Check sheet for the drawn part. Datum: minimum x, y, z corner. Units: mm. Give positions to 0.01 mm unless a question says otherwise; leave off trailing zeros. Write each loop counter-clockwise with the first axis right and the second up, starting at its lowest first coordinate (ties: lowest second). Pieces come first, ordered by that corner, then holes. Notation, with made-up numbers: (-6, 67) -> (0, 67) arc R24 ccw to (0, 102) -> close; hole circle Ø10 at (41, 49.25). An arc over 180 degrees is marked (long way). Use CSV: the item, a comma, the result in double quotes. Start each with the question number.
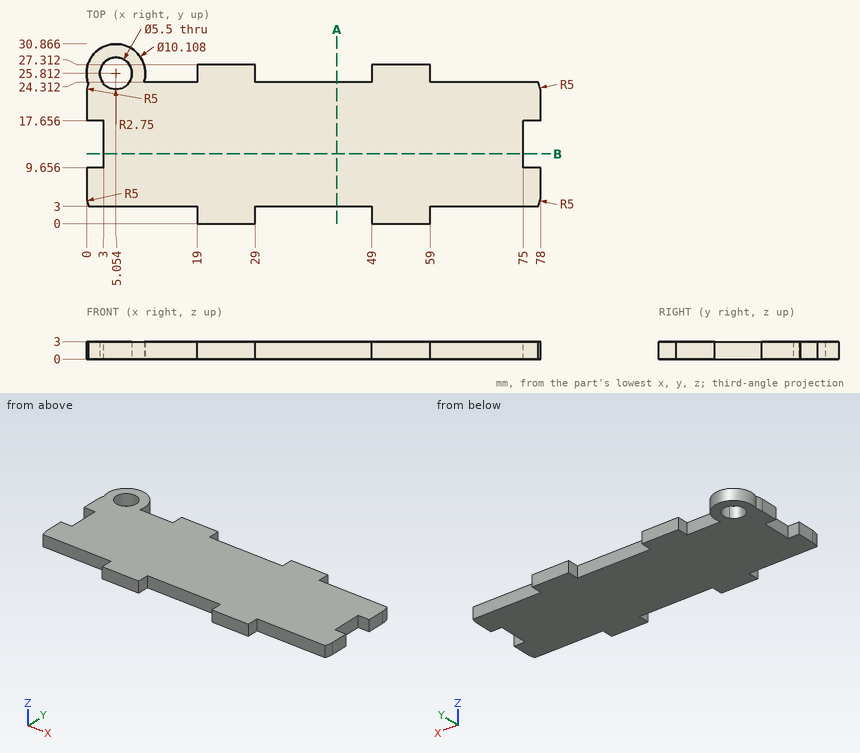
(1) Thickness scan on line 1 (Y direction, x = 64, z = 0.7); line 2 (X direction, y = 10.5, z = 1); line 3 (Y direction, x = 20, z = 0.85). Record the ranges inside material, lowest first. Write a range as from..to.
(2) Section check B-B on y = 12. Record the cut outline in (x, z).
(3) Section check A-A on x = 43. Record the cut outline in (y, z).
(4) Go/stop test with flat-tipped pins: pin 1 (0.9 mm diameter, centred on y = 1, z = 1.5, fed in from +X); pin 2 (1.5 mm diameter, centred on x = 14, z = 2, fed in from -Y). Record where each tip stops, or that it passes through.
Data:
1,line 1,"y = 3..24.31"
1,line 2,"x = 3..75"
1,line 3,"y = 0..27.31"
2,outline,"(3, 0) -> (75, 0) -> (75, 3) -> (3, 3) -> close"
3,outline,"(3, 0) -> (24.31, 0) -> (24.31, 3) -> (3, 3) -> close"
4,pin 1,"stops at x = 59"
4,pin 2,"stops at y = 3"
